Geometry: see drawing. Coordinates: mm, zero at the bounding-box minimum. Round coordinates to 2 decimals unless told otherwise and drop trailing zeros. Order: outer loops, then holes, each group sorted by start corner. A loop starts at its lowest first (then second) coordinate and runs counter-clockwise, first axis right, second up. Notation, with made-up numbers: M -35,-2.5 L -5,-2.5 A28 ccw -5,27.5 Z; hole C 2,89 d7. An arc over 180 degrees is marked long. Answer in a Markdown table with one row per item. Add a question column.
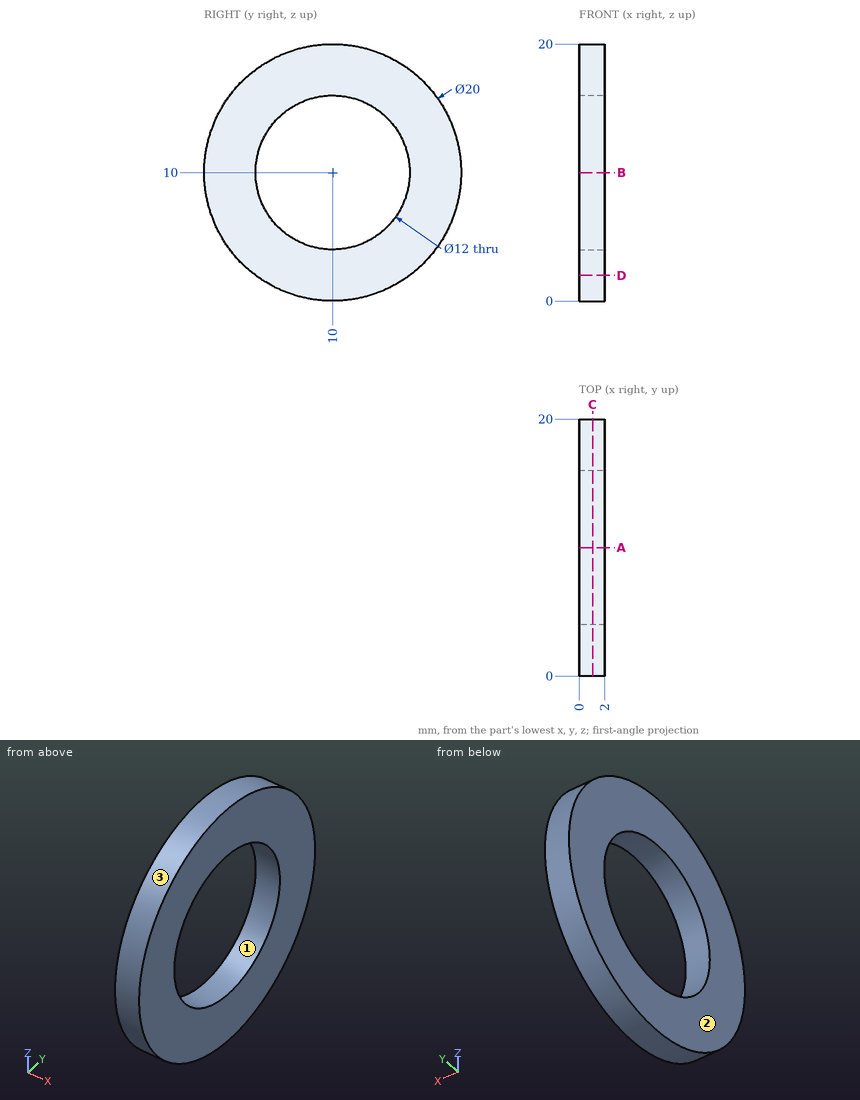
(1) Draft query along Y for the marked faces 1, 2 and 3. Return one class per face: +Y half, -Y half, draft (parallel to the pull), parting line (faces both ways), or undercut.
(2) Cut plane A-A (y = 10). Return loops of the section in (x, z), and give its area (3 significant figures).
(3) Cut plane D-D (z = 2). Return loops of the section in (x, y).
(4) Cut plane C-C (x = 1.05). Return loops of the section in (y, z).
(5) Pin query (flat end, axial travel): pin 1 (1.5 mm diameter, centred on y = 13, z = 13.5, fed in from +X). Return the tip coordinate at first contact, or that it passes through.
(6) Line query: line 1 (Z direction, x = 1.4, y = 10); line 2 (Y direction, x = 1.2, z = 12.25); line 3 (Z direction, x = 1.95, y = 6.5). Output: solid intervals per line, ascending. Write a range as from..to.
Answer list:
| question | item | result |
|---|---|---|
| 1 | face 1 | undercut |
| 1 | face 2 | draft |
| 1 | face 3 | parting line |
| 2 | outline | M 0,0 L 2,0 L 2,4 L 0,4 Z; M 0,16 L 2,16 L 2,20 L 0,20 Z |
| 2 | area | 16.0 mm² |
| 3 | outline | M 0,4 L 2,4 L 2,16 L 0,16 Z |
| 4 | outline | C 10,10 d20; hole C 10,10 d12 |
| 5 | pin 1 | through |
| 6 | line 1 | 0..4, 16..20 |
| 6 | line 2 | 0.26..4.44, 15.56..19.74 |
| 6 | line 3 | 0.63..5.13, 14.87..19.37 |
